The model under review builds one solid part; all positions refer to its coordinate system, in mm. A direction names the side the tool comes from. Round coordinates to 2 decimals unless told otherwise and drop trailing zeros. Loops run counter-clockwise (first coordinate to the right, second up) from the corner with the lowest first, then second, coordinate; pieces in that order, holes last. Notation, with made-up numbers: M 64,66 L 110,66 A4 cw 110,72 Z; hole C 44.25,1 d11. An arc over 180 degrees is marked long. Return JSON: item names as keys, results as strings. Group by question number.
Q1. Consider section A-A (z = 1.3). State the section outline as (x, y) points, and give its area (3 significant figures).
Q2. Consider section B-B (x = 748.5). State the section outline as (y, z) points.
Q3. Consider section C-C (y = 55). State the section outline as (x, z) points, and give its area (3 significant figures).
Q4. Draft analysis for pull direction Y (two halves, no side actions). For faces 1 (the face through (761.34, 72.92, 0.04)), 2 (the face through (811.602, 111.985, 0.035)), 3 (the face through (763, 55, -2.5)), state which applies: pulls with the +Y half, pulls with the -Y half, needs draft (parallel to the pull), parting line crosses it, or undercut.
Q5. For faces 4 (the face through (763, 55, 2.5)), 5 (the face through (803.232, 79.243, 0.035)), 6 (the face through (734.3, 20.2, 0)), 7 (the face through (784.712, 72.741, 0.035)), 8 (the face through (742.715, 52.904, 0.035)), list the 3-axis set-ups (+Z, -Z, +X, -X, +Y, -Y) from which the entire face can be reached by the end or side of a thin tool; tool diameter is ignored.
Q6. Clearance check with flat-ended pins moving along their axes: pin 1 Ø1.5 at (x, z) = (770.5, -1) entering from +Y; pin 2 Ø1 at (x, z) = (759, 0.5) entering from -Y; pin 3 Ø1.5 at (x, z) = (774, 0) entering from -Y; pin 4 Ø1.8 at (x, y) = (780.77, 52.57) entering from +Z. State where each tip first meets the part, or that it passes through.
Q7. Consider section D-D (x = 792.5). State the section outline as (y, z) points, and give its area (3 significant figures).
Q8. To check wall thickness, follow line 1 along X through (y, z) = (64, -1.4); line 2 along Y through (x, z) = (767, -2.2); line 3 along X through (y, z) = (70, -0.55). State the ranges of each line that lie inside material, in increasing order.
from build123d import *

# Parameters (mm, degrees)
BOSS_EXTRUDE1_DEPTH = 2.5


with BuildPart() as part:
    # Model → Boss-Extrude1 (new, symmetric)
    with BuildSketch(Plane.XY):
        with BuildLine():
            ThreePointArc((807.400029607, 115.214424851), (759.927821467, 108.213195948), (740.008452339, 64.557194238))
            ThreePointArc((740.008452339, 64.557194238), (742.783849766, 52.747710067), (749.639069353, 42.739078209))
            ThreePointArc((749.639069353, 42.739078209), (747.292156458, 25.994108012), (730.547186261, 23.647195117))
            ThreePointArc((730.547186261, 23.647195117), (734.400795358, 20.115585583), (738.547156658, 16.932779125))
            ThreePointArc((738.547156658, 16.932779125), (786.019364798, 23.934008028), (805.938733926, 67.590009739))
            ThreePointArc((805.938733926, 67.590009739), (803.163336499, 79.399493909), (796.308116912, 89.408125767))
            ThreePointArc((796.308116912, 89.408125767), (798.655029807, 106.153095964), (815.400000004, 108.500008859))
            ThreePointArc((815.400000004, 108.500008859), (811.546390907, 112.031618393), (807.400029607, 115.214424851))
        make_face()
        with BuildLine():
            Line((788.062050401, 66.939627392), (781.267821767, 78.707576584))
            ThreePointArc((781.267821767, 78.707576584), (781.267821767, 80.439627392), (779.767821767, 79.573601988))
            Line((779.767821767, 79.573601988), (765.179364498, 79.573601988))
            Line((765.179364498, 79.573601988), (757.385135864, 66.073601988))
            Line((757.385135864, 66.073601988), (765.179364498, 52.573601988))
            Line((765.179364498, 52.573601988), (779.767821767, 52.573601988))
            ThreePointArc((779.767821767, 52.573601988), (781.267821767, 51.707576584), (781.267821767, 53.439627392))
            Line((781.267821767, 53.439627392), (788.062050401, 65.207576584))
            ThreePointArc((788.062050401, 65.207576584), (789.562050401, 66.073601988), (788.062050401, 66.939627392))
        make_face(mode=Mode.SUBTRACT)
    extrude(amount=BOSS_EXTRUDE1_DEPTH, both=True)


solid = part.part
Values:
{
 "1": {"outline": "M 730.55,23.65 A60 ccw 738.55,16.93 A50.21 ccw 805.94,67.59 A33 ccw 796.31,89.41 A14.04 cw 815.4,108.5 A60 ccw 807.4,115.21 A50.21 ccw 740.01,64.56 A33 ccw 749.64,42.74 A14.04 cw Z; hole M 757.39,66.07 L 765.18,52.57 L 779.77,52.57 A1 ccw long 781.27,53.44 L 788.06,65.21 A1 ccw long 788.06,66.94 L 781.27,78.71 A1 ccw long 779.77,79.57 L 765.18,79.57 Z", "area": "4,680 mm2"},
 "2": {"outline": "M 14.4,-2.5 L 27.37,-2.5 L 27.37,2.5 L 14.4,2.5 Z; M 43.94,-2.5 L 96.2,-2.5 L 96.2,2.5 L 43.94,2.5 Z"},
 "3": {"outline": "M 741.89,-2.5 L 763.78,-2.5 L 763.78,2.5 L 741.89,2.5 Z; M 782.17,-2.5 L 805.24,-2.5 L 805.24,2.5 L 782.17,2.5 Z", "area": "225 mm2"},
 "4": {"face 1": "undercut", "face 2": "pulls with the +Y half", "face 3": "needs draft"},
 "5": {"face 4": "+Z, +X, -X, +Y, -Y", "face 5": "+Z, -Z, +X", "face 6": "+Z, -Z, -X, -Y", "face 7": "+Z, -Z", "face 8": "+Z, -Z, -X"},
 "6": {"pin 1": "stops at y = 114.62", "pin 2": "stops at y = 13.93", "pin 3": "stops at y = 16.97", "pin 4": "passes through"},
 "7": {"outline": "M 29.75,-2.5 L 118.23,-2.5 L 118.23,2.5 L 29.75,2.5 Z", "area": "442 mm2"},
 "8": {"line 1": "x = 740.04 to 758.58, 787.36 to 806.06", "line 2": "y = 15.11 to 52.57, 79.57 to 112.66", "line 3": "x = 739.92 to 759.65, 786.3 to 805.74"}
}
